Verification items for this drawing (mm, ordinates from the low corner). A direction names the side the tool comes from. Coordinates: 2 decimals unless noted, no trailing zeros. Write each loop counter-clockwise with the first axis right and the second up, starting at its lowest first coordinate (ties: lowest second). Pieces come first, ordered by that corner, then holes.
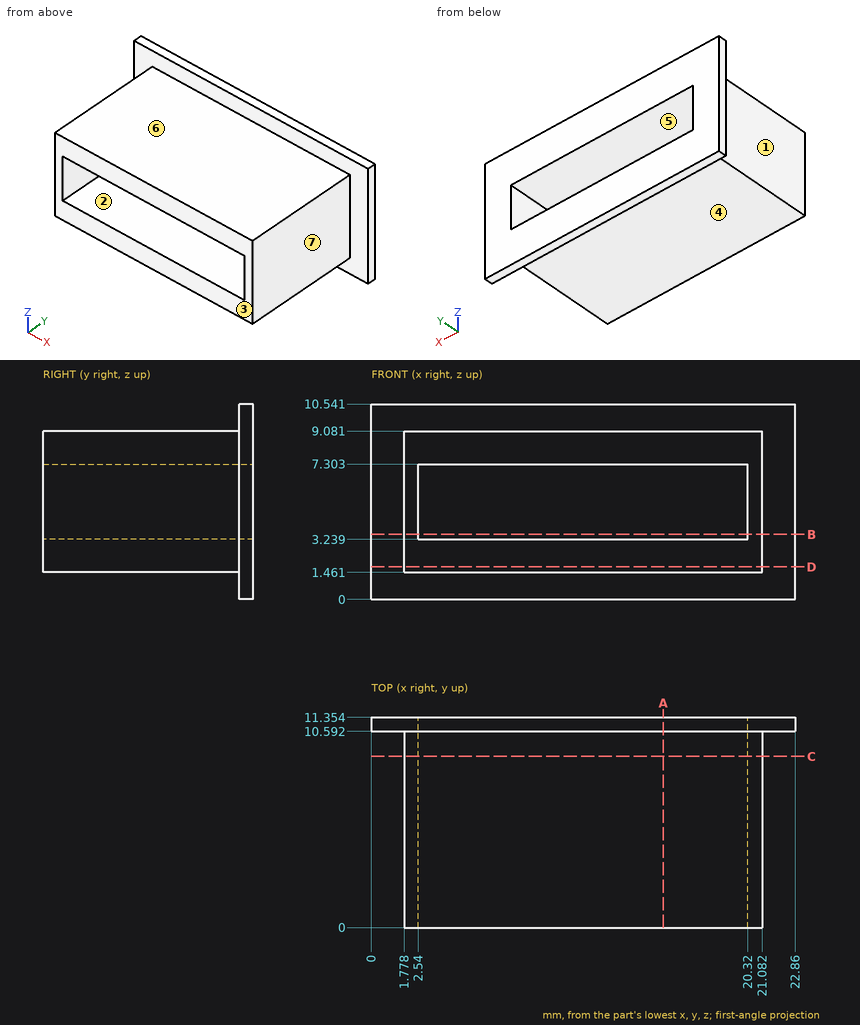
1. Thickness scan on line 1 along X through (y, z) = (8.5, 5.5); line 2 along Z through (x, y) = (3.25, 1.75); line 3 along X through (y, z) = (10.5, 7.75). Record the ranges inside material, lowest first.
Computed values:
line 1: x = 1.78 to 2.54, 20.32 to 21.08
line 2: z = 1.46 to 3.24, 7.3 to 9.08
line 3: x = 1.78 to 21.08
2. Sectioned sample at C-C, the plane y = 9.25. Record the boundary of the cut face in (x, z).
Computed values:
outline: (1.78, 1.46) - (21.08, 1.46) - (21.08, 9.08) - (1.78, 9.08) - close; hole (2.54, 3.24) - (20.32, 3.24) - (20.32, 7.3) - (2.54, 7.3) - close
3. Sectioned sample at D-D, the plane z = 1.75. Record the boundary of the cut face in (x, y), and give its area (3 significant figures).
Computed values:
outline: (0, 10.59) - (1.78, 10.59) - (1.78, 0) - (21.08, 0) - (21.08, 10.59) - (22.86, 10.59) - (22.86, 11.35) - (0, 11.35) - close
area: 222 mm2
4. Sectioned sample at A-A, the plane x = 15.75. Record the boundary of the cut face in (y, z).
Computed values:
outline: (0, 1.46) - (10.59, 1.46) - (10.59, 0) - (11.35, 0) - (11.35, 3.24) - (0, 3.24) - close; (0, 7.3) - (11.35, 7.3) - (11.35, 10.54) - (10.59, 10.54) - (10.59, 9.08) - (0, 9.08) - close
5. Access from +Z, -Z, +X, -X, +Y, -Y to the whole of each face (thin tool, end or side, straight path). Record for the marked faces 1, 2, 3 and 4.
Computed values:
face 1: +Z, -Z, -X, -Y
face 2: +Y, -Y
face 3: +Z, -Z, +X, -X, -Y
face 4: -Z, +X, -X, -Y
6. Draft check along X on the marked faces 5, 6 and 7. Enter one of: released by +X, released by -X, zero draft, split by the parting line, or undercut.
Computed values:
face 5: undercut
face 6: zero draft
face 7: released by +X
7. Sectioned sample at B-B, the plane z = 3.5. Record the boundary of the cut face in (x, y).
Computed values:
outline: (0, 10.59) - (1.78, 10.59) - (1.78, 0) - (2.54, 0) - (2.54, 11.35) - (0, 11.35) - close; (20.32, 0) - (21.08, 0) - (21.08, 10.59) - (22.86, 10.59) - (22.86, 11.35) - (20.32, 11.35) - close
8. Gauge pin test, flat ends, axial feed: pin 1 Ø1 at (x, y) = (14, 6) entering from -Z; pin 2 Ø3.5 at (y, z) = (4.5, 6) entering from +X; pin 3 Ø5.5 at (x, y) = (7.5, 6.5) entering from +Z. Record the tip position at first contact, or that the pin passes through.
Computed values:
pin 1: stops at z = 1.46
pin 2: stops at x = 21.08
pin 3: stops at z = 9.08
